```python
from build123d import *

# Parameters (mm, degrees)
CYLINDER024_R             = 13.9827
CYLINDER024_DEPTH         = 28.0162
CYLINDER023_R             = 13.9827
CYLINDER023_DEPTH         = 32.1945
FUSION011_PLACEMENT_ANGLE = 180


with BuildPart() as cylinder024:
    # Cylinder024 → Cylinder024 (new body)
    with BuildSketch(Plane.XZ.offset(-14.0081)):
        Circle(CYLINDER024_R)
    extrude(amount=CYLINDER024_DEPTH)


with BuildPart() as front_slip_l:
    # Cylinder023 → Cylinder023 (new body)
    with BuildSketch(Plane.XY):
        Circle(CYLINDER023_R)
    extrude(amount=CYLINDER023_DEPTH)

    # Fusion011: union Cylinder024
    add(cylinder024.part)


with BuildPart() as front_slip_l_1:
    # Fusion011 placement: moved
    add(front_slip_l.part.moved(Location((730.25, -50.3, 406))).rotate(Axis((730.25, -50.3, 406), (0, 1, 0)), FUSION011_PLACEMENT_ANGLE))


solid = front_slip_l_1.part
```
Work out the finished part from the listing and answer in its coordinate system (mm). A direction names the side the tool comes from. Coordinates: 2 decimals unless noted, no trailing zeros. Write each loop counter-clockwise with the first axis right and the second up, starting at its lowest first coordinate (ties: lowest second). Pieces come first, ordered by that corner, then holes.
Q1. A cutting plane is placed at B-B, the plane y = -50.3. Give the vertices of the cut face in (x, z).
Q2. A cutting plane is placed at A-A, the plane x = 739.75. Give the vertices of the cut face in (y, z), then the cut area to 3 significant figures.
Q3. Find the intervals of material crossed by line 1 (Z direction, x = 730.5, y = -61.25); line 2 (Y direction, x = 721, z = 383); line 3 (Z direction, x = 726.75, y = -56.75), in increasing order.
Q4. Each of these flat-tipped pins is pushed along its axis until it touches: pin 1 Ø3 at (y, z) = (-41, 398) entering from -X; pin 2 Ø1.5 at (y, z) = (-45.5, 380.5) entering from +X; pin 3 Ø5 at (y, z) = (-42, 396.5) entering from +X. Where does it stop, or does it pass through?
Q5. A cutting plane is placed at D-D, the plane y = -60. Give the vertices of the cut face in (x, z).
Q6. Which of the six approach directions +Z, -Z, +X, -X, +Y, -Y give full straight-line access (tool end or side, diameter ignored) to faces 1 (the face through (730, -64.308, 406)), 2 (the face through (740.556, -40.85, 386.551)), 3 (the face through (733.28, -50.1, 419.65))?
Q7. A cutting plane is placed at C-C, the plane z = 402. Give the vertices of the cut face in (x, y).
Findings below:
1. outline: (716.27, 373.81) - (744.23, 373.81) - (744.23, 406) arc R13.98 ccw to (716.27, 406) - close
2. outline: (-64.31, 395.74) - (-60.56, 395.74) - (-60.56, 373.81) - (-40.04, 373.81) - (-40.04, 395.74) - (-36.29, 395.74) - (-36.29, 416.26) - (-64.31, 416.26) - close
2. area: 1,020 mm2
3. line 1: z = 373.81 to 419.98
3. line 2: y = -60.79 to -39.81
3. line 3: z = 373.81 to 419.54
4. pin 1: stops at x = 717.87
4. pin 2: stops at x = 743.63
4. pin 3: stops at x = 742.97
5. outline: (720.18, 373.81) - (740.32, 373.81) - (740.32, 396.3) arc R13.98 ccw (long way) to (720.18, 396.3) - close
6. face 1: +Z, -Z, +X, -X, -Y
6. face 2: -Z
6. face 3: none
7. outline: (716.85, -64.31) - (743.65, -64.31) - (743.65, -54.3) arc R13.98 ccw to (743.65, -46.3) - (743.65, -36.29) - (716.85, -36.29) - (716.85, -46.3) arc R13.98 ccw to (716.85, -54.3) - close
